```python
from build123d import *

# Parameters (mm, degrees)
F0_R      = 50.8
F0_R_2    = 38.1
F1_DEPTH  = 19.05
F2_R      = 50.8
F2_R_2    = 39.37
F3_DEPTH  = 25.4
F5_DEPTH  = 12.7
F6_DEPTH  = 12.7
F7_R      = 1.9177
F8_DEPTH  = 31.75
F9_R      = 1.9177
F10_DEPTH = 31.75
F11_R     = 1.9177
F12_DEPTH = 31.75
F13_R     = 1.9177
F14_DEPTH = 31.75


with BuildPart() as f1:
    # F0 (on Right) → F1 (new body, symmetric)
    with BuildSketch(Plane.YZ):
        Circle(F0_R)
        Circle(F0_R_2, mode=Mode.SUBTRACT)
    extrude(amount=F1_DEPTH, both=True)

    # F2 (on face) → F3 (cut)
    with BuildSketch(Plane.YZ.offset(19.05)):
        Circle(F2_R)
        Circle(F2_R_2, mode=Mode.SUBTRACT)
    extrude(amount=-F3_DEPTH, mode=Mode.SUBTRACT)

    # F4 (on face) → F5 (cut)
    with BuildSketch(Plane(origin=(-19.05, 0, 0), x_dir=(0, -1, 0), z_dir=(-1, 0, 0))):
        with BuildLine():
            Line((40.560758, -2.536629), (52.733429, -2.536629))
            Line((52.733429, -2.536629), (52.733429, 2.536629))
            Line((52.733429, 2.536629), (40.560758, 2.536629))
            ThreePointArc((40.560758, 2.536629), (40.64, 0), (40.560758, -2.536629))
        make_face()
        with BuildLine():
            Line((-59.67196, -2.536629), (-40.560758, -2.536629))
            ThreePointArc((-40.560758, -2.536629), (-40.64, 0), (-40.560758, 2.536629))
            Line((-40.560758, 2.536629), (-59.67196, 2.536629))
            Line((-59.67196, 2.536629), (-59.67196, -2.536629))
        make_face()
        with BuildLine():
            Line((-2.536629, -60.94672), (2.536629, -60.94672))
            Line((2.536629, -60.94672), (2.536629, -40.560758))
            ThreePointArc((2.536629, -40.560758), (0, -40.64), (-2.536629, -40.560758))
            Line((-2.536629, -40.560758), (-2.536629, -60.94672))
        make_face()
        with BuildLine():
            Line((2.536629, 40.560758), (2.536629, 60.431999))
            Line((2.536629, 60.431999), (-2.536629, 60.431999))
            Line((-2.536629, 60.431999), (-2.536629, 40.560758))
            ThreePointArc((-2.536629, 40.560758), (0, 40.64), (2.536629, 40.560758))
        make_face()
    extrude(amount=-F5_DEPTH, mode=Mode.SUBTRACT)

    # F4 (on face) → F6 (cut)
    with BuildSketch(Plane(origin=(-19.05, 0, 0), x_dir=(0, -1, 0), z_dir=(-1, 0, 0))):
        with BuildLine():
            Line((40.560758, -2.536629), (52.733429, -2.536629))
            Line((52.733429, -2.536629), (52.733429, 2.536629))
            Line((52.733429, 2.536629), (40.560758, 2.536629))
            ThreePointArc((40.560758, 2.536629), (40.64, 0), (40.560758, -2.536629))
        make_face()
        with BuildLine():
            Line((-59.67196, -2.536629), (-40.560758, -2.536629))
            ThreePointArc((-40.560758, -2.536629), (-40.64, 0), (-40.560758, 2.536629))
            Line((-40.560758, 2.536629), (-59.67196, 2.536629))
            Line((-59.67196, 2.536629), (-59.67196, -2.536629))
        make_face()
        with BuildLine():
            Line((-2.536629, -60.94672), (2.536629, -60.94672))
            Line((2.536629, -60.94672), (2.536629, -40.560758))
            ThreePointArc((2.536629, -40.560758), (0, -40.64), (-2.536629, -40.560758))
            Line((-2.536629, -40.560758), (-2.536629, -60.94672))
        make_face()
        with BuildLine():
            Line((2.536629, 40.560758), (2.536629, 60.431999))
            Line((2.536629, 60.431999), (-2.536629, 60.431999))
            Line((-2.536629, 60.431999), (-2.536629, 40.560758))
            ThreePointArc((-2.536629, 40.560758), (0, 40.64), (2.536629, 40.560758))
        make_face()
    extrude(amount=-F6_DEPTH, mode=Mode.SUBTRACT)

    # F7 (on face) → F8 (cut, symmetric)
    with BuildSketch(Plane(origin=(0, 0, 2.536629), x_dir=(1, 0, 0), z_dir=(0, 0, -1))):
        with Locations((-12.7, 44.37585)):
            Circle(F7_R)
    extrude(amount=F8_DEPTH, both=True, mode=Mode.SUBTRACT)

    # F9 (on face) → F10 (cut, symmetric)
    with BuildSketch(Plane.XY.offset(-2.536629)):
        with Locations((-12.7, 44.37585)):
            Circle(F9_R)
    extrude(amount=F10_DEPTH, both=True, mode=Mode.SUBTRACT)

    # F11 (on face) → F12 (cut, symmetric)
    with BuildSketch(Plane.XZ.offset(-2.536629)):
        with Locations((-12.7, 44.37585)):
            Circle(F11_R)
    extrude(amount=F12_DEPTH, both=True, mode=Mode.SUBTRACT)

    # F13 (on face) → F14 (cut, symmetric)
    with BuildSketch(Plane(origin=(0, -2.536629, 0), x_dir=(-1, 0, 0), z_dir=(0, 1, 0))):
        with Locations((12.7, -44.37585)):
            Circle(F13_R)
    extrude(amount=F14_DEPTH, both=True, mode=Mode.SUBTRACT)


solid = f1.part
```
Model file for the job. Use its own axes, mm. A direction names the side the tool comes from. Coordinates: 2 decimals unless noted, no trailing zeros. Order: outer loops, then holes, each group sorted by start corner. A loop starts at its lowest first (then second) coordinate and runs counter-clockwise, first axis right, second up. Notation, with made-up numbers: (-31.5, 76.5) - (-2.5, 76.5) arc R28 cw to (-2.5, 115.5) - close; hole circle Ø4 at (-31.5, -27.5). An arc over 180 degrees is marked (long way). Return JSON: item names as keys, results as strings. Group by question number.
1) Saw through at D-D, the plane y = -13.5. Write the cut outline in (x, z).
2) Probe line 1 (Z direction, x = -13, y = -9); line 2 (Z direction, x = -11.5, y = 0); line 3 (Z direction, x = 10.5, y = 0). List the from-to ranges inside material, lowest first. Write a range as from..to.
3) Mould opens along Y. For faces 6 (the cylindrical face through (-12.79, -40.64, 0.04)), 7 (the cylindrical face through (-12.79, -0.04, -40.64)), 8 (the flat face through (19.05, -21, 32)) say: released by +Y, released by -Y, zero draft, split by the parting line, or undercut.
4) Tool access for faces 1 (the flat face through (-13, -47, 2.537)), 2 (the flat face through (-6.35, -12, 38)), 3 (the flat face through (-13, 2.537, -47)), 4 (the flat face through (-13, 47, 2.537)), 5 (the flat face through (-13, -2.537, 47)): list every direction of +Z, -Z, +X, -X, +Y, -Y with a clear straight run to the whole face (end or side of a thin tool).
5) Flat gauge pins, fed straight in: P1, Ø1, axis at x = 7.5, z = 10.5, coming from the -Y side; P2, Ø5, axis at x = -13.5, z = 46.5, coming from the +Y side; P3, Ø2, axis at x = 4.5, y = -35, coming from the +Z side; P4, Ø3.5, axis at x = -12.7, y = 44.38, coming from the -Z side. Where does each tip first touch, or does it go through?
6) Saw through at B-B, the plane x = -8.5. Write the cut outline in (y, z).
7) Saw through at A-A, the plane y = 0. Write the cut outline in (x, z).
Values found:
{
 "1": {"outline": "(-19.05, -48.97) - (-6.35, -48.97) - (-6.35, -36.98) - (19.05, -36.98) - (19.05, -35.63) - (-19.05, -35.63) - close; (-19.05, 35.63) - (19.05, 35.63) - (19.05, 36.98) - (-6.35, 36.98) - (-6.35, 48.97) - (-19.05, 48.97) - close; hole circle Ø3.84 at (-12.7, -44.38); hole circle Ø3.84 at (-12.7, 44.38)"},
 "2": {"line 1": "z = -50..-46.27, -42.48..-37.02, 37.02..42.48, 46.27..50", "line 2": "z = -40.64..-38.1, 38.1..40.64", "line 3": "z = -39.37..-38.1, 38.1..39.37"},
 "3": {"face 6": "released by -Y", "face 7": "undercut", "face 8": "zero draft"},
 "4": {"face 1": "+X, -X, -Y", "face 2": "+X", "face 3": "-Z, +X, -X", "face 4": "+X, -X, +Y", "face 5": "+Z, +X, -X"},
 "5": {"P1": "stops at y = -38.08", "P2": "stops at y = 24.93", "P3": "stops at z = 19.85", "P4": "passes through"},
 "6": {"outline": "(-50.74, -2.54) arc R50.8 ccw to (-2.54, -50.74) - (-2.54, -40.56) arc R40.64 ccw to (2.54, -40.56) - (2.54, -50.74) arc R50.8 ccw to (50.74, -2.54) - (40.56, -2.54) arc R40.64 ccw to (40.56, 2.54) - (50.74, 2.54) arc R50.8 ccw to (2.54, 50.74) - (2.54, 40.56) arc R40.64 ccw to (-2.54, 40.56) - (-2.54, 50.74) arc R50.8 ccw to (-50.74, 2.54) - (-40.56, 2.54) arc R40.64 ccw to (-40.56, -2.54) - close; hole circle Ø76.2 at (0, 0)"},
 "7": {"outline": "(-19.05, -40.64) - (-6.35, -40.64) - (-6.35, -39.37) - (19.05, -39.37) - (19.05, -38.1) - (-19.05, -38.1) - close; (-19.05, 38.1) - (19.05, 38.1) - (19.05, 39.37) - (-6.35, 39.37) - (-6.35, 40.64) - (-19.05, 40.64) - close"}
}
